Can you work these out from the model? Positions are in its coordinate system, mm. A direction names the side the tool comes from. Coordinates: 2 decimals unless noted, no trailing zeros. Loops run counter-clockwise (first coordinate to the right, second up) from the corner with the lowest first, then second, coordinate; pieces in that order, holes last. Notation, with made-up numbers: (83, 10.5) -> (138, 10.5) arc R20 ccw to (138, 14.5) -> close; hole circle Ø9 at (-28.5, -17). An arc over 180 degrees is marked (long way). Put each result on its own line as item: value. Start each with the question number.
Item 1: Please list where these lines run through material, in increasing order: L1, parallel to X at y = 0.85, z = 1.25; L2, parallel to Z at x = 0.5, y = 2; L3, parallel to Z at x = -0.6, y = 1. Write a range as from..to.
Item 2: If we section it at C-C on z = 0.5: Please give me the cut outline in (x, y).
Item 3: If we section it at A-A on y = 2.4: Please give me the cut outline in (x, z).
Item 4: For faces 1 (the flat face through (0, 1, -6.651)), 2 (the cylindrical face through (0.36, 1.52, 8.35)), which set-ups out of +Z, -Z, +X, -X, +Y, -Y let a thin tool reach every point of the face, with its end or its side?
Item 5: We'd pull the mould along X, two halves only. Please class faces 3 (the flat face through (2.891, 1, 1)), 4 (the flat face through (-2.109, 1, 1)), 5 (the flat face through (2.1, 3, 1.5)), 6 (the flat face through (1.891, 2, 1)): pulls with the +X half, pulls with the -X half, needs draft (parallel to the pull), parting line crosses it, or undercut.
Item 6: If we section it at B-B on x = -0.55: Please give me the cut outline in (y, z).
Autodesk Inventor part; units mm, degrees
ref_plane "YZ Plane" through (0, 0, 0) normal (1, 0, 0) x (0, 1, 0)
ref_plane "XZ Plane" through (0, 0, 0) normal (0, 1, 0) x (-1, 0, 0)
ref_plane "XY Plane" through (0, 0, 0) normal (0, 0, 1) x (1, 0, 0)
sketch "スケッチ1" plane through (0, 0, 0) normal (0, 0, 1) x (1, 0, 0)
  point P0 (0, 0)
sketch "スケッチ2" plane through (0, 0, 0) normal (0, 1, 0) x (-1, 0, 0)
  line L0 (2.109, 9.3486) -> (-2.891, 9.3486)
  line L1 (-2.891, 9.3486) -> (-2.891, -6.6514)
  line L2 (-2.891, -6.6514) -> (2.109, -6.6514)
  line L3 (2.109, -6.6514) -> (2.109, 9.3486)
  point P0 (0, 0)
  dimension "d0" = 5
  dimension "d1" = 16
extrude "押し出し1" add sketch "スケッチ2" along normal blind 3
sketch "スケッチ3" plane through (0, 3, 0) normal (0, 1, 0) x (1, 0, 0)
  line L0 (0.391, -6.8486) -> (0.391, 4.1514) construction
  line L1 (1.891, -6.8486) -> (1.891, 4.1514)
  line L2 (-1.109, 4.1514) -> (-1.109, -6.8486)
  arc A0 (-1.109, -6.8486) -> (1.891, -6.8486) centre (0.391, -6.8486) ccw
  arc A1 (1.891, 4.1514) -> (-1.109, 4.1514) centre (0.391, 4.1514) ccw
  line L3 (-2.109, 6.6514) -> (-2.109, -9.3486)
  line L4 (-2.109, -9.3486) -> (2.891, -9.3486)
  point P0 (0, 0)
  point P1 (0.391, -1.3486)
  dimension "d4" = 11
  dimension "d5" = 3
  dimension "d6" = 1
  dimension "d7" = 2.5
extrude "押し出し2" cut sketch "スケッチ3" against normal blind 3
properties part number "creat10"
Solutions:
1. L1: -2.11..-1.11, 1.89..2.89
1. L2: -6.65..-5.65, 8.34..9.35
1. L3: -6.65..-5.28, 7.97..9.35
2. outline: (-2.11, 0) -> (-1.11, 0) -> (-1.11, 3) -> (-2.11, 3) -> close; (1.89, 0) -> (2.89, 0) -> (2.89, 3) -> (1.89, 3) -> close
3. outline: (-2.11, -6.65) -> (2.89, -6.65) -> (2.89, 9.35) -> (-2.11, 9.35) -> close; hole (-1.11, -4.15) arc R1.5 ccw to (1.89, -4.15) -> (1.89, 6.85) arc R1.5 ccw to (-1.11, 6.85) -> close
4. face 1: -Z, +X, -X, +Y, -Y
4. face 2: +Y, -Y
5. face 3: pulls with the +X half
5. face 4: pulls with the -X half
5. face 5: needs draft
5. face 6: undercut
6. outline: (0, -6.65) -> (3, -6.65) -> (3, -5.32) -> (0, -5.32) -> close; (0, 8.02) -> (3, 8.02) -> (3, 9.35) -> (0, 9.35) -> close
